Input: part model. Units: mm. Frame: model coordinates. Face numbers are marked on the shaded views. Give positions to 0.01 mm unless a question says otherwise; leave off trailing zeros. Write each loop counter-clockwise with the first axis right and the second up, starting at its lowest first coordinate (ties: lowest second). Pieces come first, ordered by that corner, then holes.
```python
from build123d import *

# Parameters (mm, degrees)
BODY_DEPTH = 0.635


with BuildPart() as part:
    # BodySke → Body (new body)
    with BuildSketch(Plane.XY):
        with BuildLine():
            Line((3.08825445, -3.08825445), (2.375594962, -3.08825445))
            ThreePointArc((2.375594962, -3.08825445), (1.700235197, -2.808511276), (1.420492024, -2.133151512))
            Line((1.420492024, -2.133151512), (1.420492024, -0.400356828))
            ThreePointArc((1.420492024, -0.400356828), (1.442066538, -0.348271343), (1.494152024, -0.326696828))
            Line((1.494152024, -0.326696828), (3.080912536, -0.326696828))
            ThreePointArc((3.080912536, -0.326696828), (3.392132841, -0.166234942), (3.441920608, 0.180358874))
            ThreePointArc((3.441920608, 0.180358874), (2.530552339, 1.608327553), (1.071838527, 2.46962929))
            ThreePointArc((1.071838527, 2.46962929), (0.774531372, 2.438826913), (0.590394611, 2.203382686))
            Line((0.590394611, 2.203382686), (0.381292217, 1.423001927))
            ThreePointArc((0.381292217, 1.423001927), (0, 1.4732), (-0.381292217, 1.423001927))
            Line((-0.381292217, 1.423001927), (-0.590394611, 2.203382686))
            ThreePointArc((-0.590394611, 2.203382686), (-0.774531372, 2.438826913), (-1.071838527, 2.46962929))
            ThreePointArc((-1.071838527, 2.46962929), (-2.530552339, 1.608327553), (-3.441920608, 0.180358874))
            ThreePointArc((-3.441920608, 0.180358874), (-3.392132841, -0.166234942), (-3.080912536, -0.326696828))
            Line((-3.080912536, -0.326696828), (-1.494152024, -0.326696828))
            ThreePointArc((-1.494152024, -0.326696828), (-1.442066538, -0.348271343), (-1.420492024, -0.400356828))
            Line((-1.420492024, -0.400356828), (-1.420492024, -2.133151512))
            ThreePointArc((-1.420492024, -2.133151512), (-1.700235197, -2.808511276), (-2.375594962, -3.08825445))
            Line((-2.375594962, -3.08825445), (-3.08825445, -3.08825445))
            ThreePointArc((-3.08825445, -3.08825445), (0, 4.367451327), (3.08825445, -3.08825445))
        make_face()
    extrude(amount=-BODY_DEPTH)


solid = part.part
```
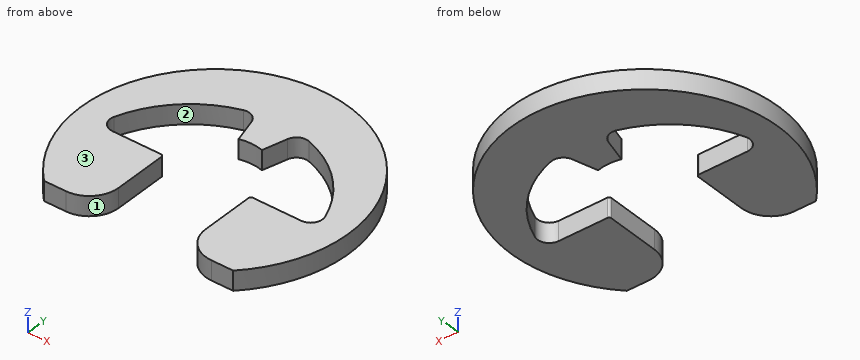
Item 1: Section D-D (x = 0). Return loops of the section in (y, z) (3 decimals).
Item 2: Mould query, pull axis Y, two halves, no side actions, for the marked faces 1, 2 and 3. Classes: +Y half, -Y half, draft (parallel to the pull), parting line (faces both ways), or undercut.
Item 3: Section A-A (z = -0.1). Return loops of the section in (x, y).
Item 4: Section B-B (x = -2.25). Return loops of the section in (y, z) (3 decimals), and give its area (3 significant figures).
Item 5: Ray query, line 1 (X direction, y = -1, z = -0.15); line 2 (Y direction, x = 3, z = -0.45); line 3 (Y direction, x = -3.25, z = -0.25). Return the intervals inside material, ascending.
Item 6: Section C-C (y = 0). Return loops of the section in (x, z) (3 decimals), and give its area (3 significant figures).
Solved:
1. outline: (1.473, -0.635) - (4.367, -0.635) - (4.367, 0) - (1.473, 0) - close
2. face 1: -Y half
2. face 2: undercut
2. face 3: draft
3. outline: (-3.44, 0.18) arc R3.64 cw to (-1.07, 2.47) arc R0.38 cw to (-0.59, 2.2) - (-0.38, 1.42) arc R1.47 cw to (0.38, 1.42) - (0.59, 2.2) arc R0.38 cw to (1.07, 2.47) arc R3.64 cw to (3.44, 0.18) arc R0.38 cw to (3.08, -0.33) - (1.49, -0.33) arc R0.07 ccw to (1.42, -0.4) - (1.42, -2.13) arc R0.96 ccw to (2.38, -3.09) - (3.09, -3.09) arc R4.37 ccw (long way) to (-3.09, -3.09) - (-2.38, -3.09) arc R0.96 ccw to (-1.42, -2.13) - (-1.42, -0.4) arc R0.07 ccw to (-1.49, -0.33) - (-3.08, -0.33) arc R0.38 cw to start
4. outline: (-3.08, -0.635) - (-0.327, -0.635) - (-0.327, 0) - (-3.08, 0) - close; (1.853, -0.635) - (3.743, -0.635) - (3.743, 0) - (1.853, 0) - close
4. area: 2.95 mm2
5. line 1: x = -4.25 to -1.42, 1.42 to 4.25
5. line 2: y = -3.09 to -0.33, 1.05 to 3.17
5. line 3: y = -2.92 to -0.29, 0.63 to 2.92
6. outline: (-4.367, -0.635) - (-3.459, -0.635) - (-3.459, 0) - (-4.367, 0) - close; (3.459, -0.635) - (4.367, -0.635) - (4.367, 0) - (3.459, 0) - close
6. area: 1.15 mm2
